Can you work these out from the model? Positions are in its coordinate system, mm. Face numbers are marked on the shaded views. Give positions to 0.01 mm unless a question says otherwise; leave off trailing zeros. Write each loop counter-clockwise with the first axis right and the second up, starting at its lowest first coordinate (ties: lowest second). Pieces come first, ordered by that corner, then holes. Notation, with made-up numbers: M 10.25,-2 L 58.25,-2 A28 cw 58.25,31 Z; hole C 13.5,-23 d6. An arc over 180 degrees is marked long. Write each question's results on one line, items separated by ' | '.
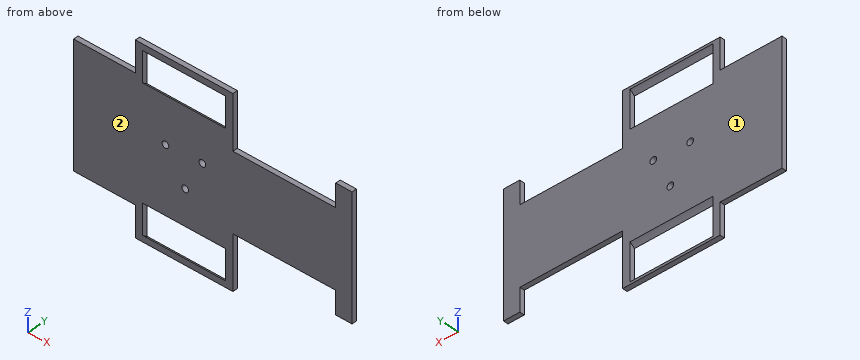
from build123d import *

# Parameters (mm, degrees)
BOSS_EXTRUDE1_DEPTH    = 4
SPLIT2_SURFACE_1_BACK  = 275.772
SPLIT2_SURFACE_1_DEPTH = 551.544
SPLIT2_SURFACE_2_BACK  = 275.772
SPLIT2_SURFACE_2_DEPTH = 551.544
BOSS_EXTRUDE4_START    = -76.2
BOSS_EXTRUDE4_DEPTH    = 152.4
SKETCH8_R              = 17.5
CUT_EXTRUDE4_DEPTH     = 68
SKETCH11_R             = 2.75
CUT_EXTRUDE6_DEPTH     = 138.734999183
SKETCH12_W             = 167.624585895
SKETCH12_H             = 26.062825832
CUT_EXTRUDE7_DEPTH     = 147.892749991


with BuildPart() as part:
    # Sketch1 → Boss-Extrude1 (new body)
    with BuildSketch(Plane(origin=(0, 0, 0), x_dir=(1, 0, 0), z_dir=(0, 1, 0))):
        Polygon((-114.3, 50.8), (-114.3, -50.8), (-63.5, -50.8), (-63.5, -76.2), (16.5, -76.2), (16.5, -31.75), (100.867964722, -31.75), (100.867964722, -50.8), (114.3, -50.8), (114.3, 50.8), (100.867964722, 50.8), (100.867964722, 31.75), (16.5, 31.75), (16.5, 76.2), (-63.5, 76.2), (-63.5, 50.8), align=None)
    extrude(amount=BOSS_EXTRUDE1_DEPTH)


with BuildPart() as body_2:
    # Split2: the piece behind the surface
    add(part.part)
    # Split2 surface: a surface, the sketch's curves swept straight by 551.544 mm
    with BuildLine(Plane.XY.offset(76.2).offset(-SPLIT2_SURFACE_1_BACK), mode=Mode.PRIVATE) as split2_surface_1_path:
        Line((16.5, 0), (-23.5, 0))
        Line((-23.5, 0), (-23.5, 2))
        Line((-23.5, 2), (-63.5, 2))
        Line((-63.5, 2), (-63.5, 4))
    split2_surface_1 = Shell.extrude(split2_surface_1_path.wire(), (0 * SPLIT2_SURFACE_1_DEPTH, 0 * SPLIT2_SURFACE_1_DEPTH, 1 * SPLIT2_SURFACE_1_DEPTH))
    split(bisect_by=split2_surface_1, keep=Keep.BOTTOM)


with BuildPart() as part_1:
    add(part.part)

    # Split2: split by a surface, the side it looks to stays
    # Split2 surface: a surface, the sketch's curves swept straight by 551.544 mm
    with BuildLine(Plane.XY.offset(76.2).offset(-SPLIT2_SURFACE_2_BACK), mode=Mode.PRIVATE) as split2_surface_2_path:
        Line((16.5, 0), (-23.5, 0))
        Line((-23.5, 0), (-23.5, 2))
        Line((-23.5, 2), (-63.5, 2))
        Line((-63.5, 2), (-63.5, 4))
    split2_surface_2 = Shell.extrude(split2_surface_2_path.wire(), (0 * SPLIT2_SURFACE_2_DEPTH, 0 * SPLIT2_SURFACE_2_DEPTH, 1 * SPLIT2_SURFACE_2_DEPTH))
    split(bisect_by=split2_surface_2, keep=Keep.TOP)

    add(body_2.part)  # Boss-Extrude4 merges body 2
    # Boss-Extrude4: read off the stored shape, not the designer's step
    # Boss-Extrude4 outline → Boss-Extrude4 (add)
    with BuildSketch(Plane.XY.offset(BOSS_EXTRUDE4_START)):
        Polygon((-57.5, 4), (-63.5, 4), (-63.5, 0), (16.5, 0), (16.5, 4), (10.5, 4), (10.5, 14), (-57.5, 14), align=None)
    extrude(amount=BOSS_EXTRUDE4_DEPTH)

    # Sketch8 → Cut-Extrude4 (cut)
    with BuildSketch(Plane(origin=(10.5, 0, 0), x_dir=(0, 0, -1), z_dir=(1, 0, 0))):
        with Locations((-58.7, 12.344512168)):
            Circle(SKETCH8_R)
        with Locations((58.7, 12.344512168)):
            Circle(SKETCH8_R)
    extrude(amount=-CUT_EXTRUDE4_DEPTH, mode=Mode.SUBTRACT)


with BuildPart() as cut_extrude4_piece_1:
    # of the separate pieces the step leaves, piece 1, a body of its own (cut_extrude4_pieces)
    add(part_1.part.solids().sort_by_distance((16.5, 0, -31.75))[0])

    # Sketch11 → Cut-Extrude6 (cut, through all)
    with BuildSketch(Plane(origin=(0, 4, 0), x_dir=(1, 0, 0), z_dir=(0, 1, 0))):
        with Locations(Location((-22.643612575, 17.341502836, 0), (0, 0, 270))):
            Circle(SKETCH11_R)
        with Locations(Location((-38.877222753, -8.255760701, 0), (0, 0, 270))):
            Circle(SKETCH11_R)
        with Locations(Location((-8.592537174, -9.515847743, 0), (0, 0, 270))):
            Circle(SKETCH11_R)
    extrude(amount=-CUT_EXTRUDE6_DEPTH, mode=Mode.SUBTRACT)


with BuildPart() as cut_extrude4_piece_2:
    # of the separate pieces the step leaves, piece 2, a body of its own (cut_extrude4_pieces)
    add(part_1.part.solids().sort_by_distance((10.5, 14, 76.2))[0])


with BuildPart() as cut_extrude4_piece_3:
    # of the separate pieces the step leaves, piece 3, a body of its own (cut_extrude4_pieces)
    add(part_1.part.solids().sort_by_distance((-57.5, 14, -76.2))[0])


with BuildPart() as cut_extrude7_tool:
    # Sketch12 → Cut-Extrude7 (new, through all)
    with BuildSketch(Plane(origin=(10.5, 0, 0), x_dir=(0, 0, -1), z_dir=(1, 0, 0))):
        with Locations((1.392837232, 17.031412916)):
            Rectangle(SKETCH12_W, SKETCH12_H)
    extrude(amount=-CUT_EXTRUDE7_DEPTH)


with BuildPart() as cut_extrude4_piece_1_1:
    add(cut_extrude4_piece_1.part)

    # Cut-Extrude7: cut by cut_extrude7_tool
    add(cut_extrude7_tool.part, mode=Mode.SUBTRACT)


with BuildPart() as cut_extrude4_piece_2_1:
    add(cut_extrude4_piece_2.part)

    # Cut-Extrude7: cut by cut_extrude7_tool
    add(cut_extrude7_tool.part, mode=Mode.SUBTRACT)


with BuildPart() as cut_extrude4_piece_3_1:
    add(cut_extrude4_piece_3.part)

    # Cut-Extrude7: cut by cut_extrude7_tool
    add(cut_extrude7_tool.part, mode=Mode.SUBTRACT)


solid = cut_extrude4_piece_1_1.part
Item 1: I want a section at D-D, the plane x = 75. Please give me the cut outline in (y, z).
Geometry says:
outline: M 0,-31.75 L 4,-31.75 L 4,31.75 L 0,31.75 Z
Item 2: I want a section at B-B, the plane x = -30.5. Please give me the cut outline in (y, z).
Geometry says:
outline: M 0,-76.2 L 4,-76.2 L 4,-74.08 A17.5 cw 0,-71.1 Z; M 0,-46.3 A17.5 cw 4,-43.32 L 4,43.32 A17.5 cw 0,46.3 Z; M 0,71.1 A17.5 cw 4,74.08 L 4,76.2 L 0,76.2 Z
Item 3: I'm going to push flat-ended pins straight in: pin 1 (3.5 mm diameter, centred on x = -22.64, z = -17.34, fed in from -Y); pin 2 (2 mm diameter, centred on x = 108, y = 1.5, fed in from +Z); pin 3 (1 mm diameter, centred on x = 35.5, y = 3.5, fed in from -Z); pin 4 (2 mm diameter, centred on x = 18, y = 3.5, fed in from +Z). Where does each tip first touch, or does it pass through?
Geometry says:
pin 1: passes through | pin 2: stops at z = 50.8 | pin 3: stops at z = -31.75 | pin 4: stops at z = 31.75
Item 4: If I drill on line 1 (X direction, y = 2.3, z = -47); line 2 (X direction, y = 1.7, z = 35.5); line 3 (X direction, y = 1.65, z = 8.5), over which ranges is the centre line in solid material (lowest first)? Write a range as from..to.
Geometry says:
line 1: x = -114.3..-57.5, 10.5..16.5, 100.87..114.3 | line 2: x = -114.3..16.5, 100.87..114.3 | line 3: x = -114.3..-41.62, -36.14..-11.15, -6.04..114.3
Item 5: I want a section at C-C, the plane y = 2.4. Please give me the cut outline in (x, z).
Geometry says:
outline: M -114.3,-50.8 L -63.5,-50.8 L -63.5,-76.2 L 16.5,-76.2 L 16.5,-31.75 L 100.87,-31.75 L 100.87,-50.8 L 114.3,-50.8 L 114.3,50.8 L 100.87,50.8 L 100.87,31.75 L 16.5,31.75 L 16.5,76.2 L -63.5,76.2 L -63.5,50.8 L -114.3,50.8 Z; hole M -57.5,-73.1 L 10.5,-73.1 L 10.5,-44.3 L -57.5,-44.3 Z; hole M -57.5,44.3 L 10.5,44.3 L 10.5,73.1 L -57.5,73.1 Z; hole C -38.88,8.26 d5.5; hole C -22.64,-17.34 d5.5; hole C -8.59,9.52 d5.5
Item 6: I want a section at A-A, the plane z = 67.5. Please give me the cut outline in (x, y).
Geometry says:
outline: M -63.5,0 L -57.5,0 L -57.5,4 L -63.5,4 Z; M 10.5,0 L 16.5,0 L 16.5,4 L 10.5,4 Z
Item 7: Thinking about a two-plate mould opening in Y: for the marked faces 1 and 2, which applies, +Y half, -Y half, draft (parallel to the pull), parting line (faces both ways), or undercut?
Geometry says:
face 1: +Y half | face 2: -Y half
